Design review of the part built by this model. Coordinates are the model's own, in mm. A direction names the side the tool comes from. Round coordinates to 2 decimals unless told otherwise and drop trailing zeros. Loops run counter-clockwise (first coordinate to the right, second up) from the corner with the lowest first, then second, coordinate; pieces in that order, holes last. Notation, with made-up numbers: (23.25, 48) -> (78.25, 48) arc R28 ccw to (78.25, 72) -> close; hole circle Ø5 at (37.5, 75). An arc over 180 degrees is marked (long way). Use a Markdown table: item, result. Add a question column.
from build123d import *

# Parameters (mm, degrees)
SKETCH_1_W                   = 25
SKETCH_1_H                   = 12
SKETCH_1_W_2                 = 21
SKETCH_1_H_2                 = 8
EXTRUDE_1_DEPTH              = 9
CUT_EXTRUDE_1_DEPTH          = 10
CHAMFER_1_SIZE               = 7
CHAMFER_1_SIZE2              = 1.875644347
HOLE_WIZARD_2_561_AT_2_COUNT = 2
HOLE_WIZARD_2_561_AT_2_PITCH = 5


with BuildPart() as part:
    # Эскиз1 → Бобышка-Вытянуть1 (new body)
    with BuildSketch(Plane.XY):
        with Locations((12.5, 6)):
            Rectangle(SKETCH_1_W, SKETCH_1_H)
        with Locations((12.5, 6)):
            Rectangle(SKETCH_1_W_2, SKETCH_1_H_2, mode=Mode.SUBTRACT)
    extrude(amount=EXTRUDE_1_DEPTH)

    # Эскиз2 → Вырез-Вытянуть1 (cut, through all)
    with BuildSketch(Plane.XY.offset(9)):
        Polygon((18, 10), (18, 12), (0, 12), (0, 0), (19, 0), (19, 2), (2, 2), (2, 10), align=None)
    extrude(amount=-CUT_EXTRUDE_1_DEPTH, mode=Mode.SUBTRACT)

    # Фаска1
    chamfer_1_edges = [part.edges().sort_by_distance(p)[0] for p in [
        (18, 11, 9),
    ]]
    chamfer_1_side = [part.faces().sort_by_distance(p)[0] for p in [
        (18, 11, 4.5),
    ]]
    chamfer(chamfer_1_edges, length=CHAMFER_1_SIZE, length2=CHAMFER_1_SIZE2, reference=chamfer_1_side[0])

    # Эскиз5 → Отверстие обработанное метчиком #2-561 (revolve, cut)
    with BuildSketch(Plane(origin=(21, 0, 2), x_dir=(0, 0, -1), z_dir=(1, 0, 0))):
        Polygon((0, 0), (0, 2), (1.27, 2), (1.0922, 1.8755031), (1.0922, 0.1244969), (1.27, 0), align=None)
    hole_wizard_2_561 = revolve(axis=Axis((21, -6.35, 2), (0, 1, 0)), mode=Mode.SUBTRACT)

    # Отверстие обработанное метчиком #2-561 at 2: Отверстие обработанное метчиком #2-561 ×2
    with Locations(*[(0, 0, i * HOLE_WIZARD_2_561_AT_2_PITCH) for i in range(1, HOLE_WIZARD_2_561_AT_2_COUNT)]):
        add(hole_wizard_2_561, mode=Mode.SUBTRACT)

    # Эскиз6 → Отверстие обработанное метчиком #2-562 (revolve, cut)
    with BuildSketch(Plane(origin=(20.222787252, 12, 4.5), x_dir=(0, 0, 1), z_dir=(1, 0, 0))):
        Polygon((0, 0), (0, 2), (1.27, 2), (1.0922, 1.8755031), (1.0922, 0.1244969), (1.27, 0), align=None)
    revolve(axis=Axis((20.222787252, 18.35, 4.5), (0, -1, 0)), mode=Mode.SUBTRACT)


solid = part.part
1. To check wall thickness, follow probe 1 along Z at (x, y) = (21, 0.85); probe 2 along Y at (x, z) = (19.75, 7.25); probe 3 along X at (y, z) = (1.2, 2). State the ranges of each line that lie inside material, in increasing order. Write a range as from..to.
2. Insertion check: P1, Ø1.5, axis at y = 7.5, z = 3, coming from the -X side; P2, Ø2, axis at y = 1.5, z = 3, coming from the -X side. Each pin has a flat end and moves straight along its axis. Give the tip position at first contact, or say it passes through.
3. Consider section C-C on x = 20.5. Give the number of separate pieces and of enclosed holes in the cut face, plus the area to 3 significant figures.
4. For faces 1 (the face through (21, 10, 3)), 2 (the face through (19, 1, 5)), 3 (the face through (22.066, 0.988, 2.237)), 4 (the face through (22, 12, 4)), 5 (the face through (18.95, 10.99, 5.55)), list the 3-axis set-ups (+Z, -Z, +X, -X, +Y, -Y) from which the entire face can be reached by the end or side of a thin tool; tool diameter is ignored.
5. Consider section D-D on z = 7. State the section outline as (x, y) points.
6. Consider section B-B on y = 9.25. State the section outline as (x, z) points, plus the area to 3 significant figures.
7. Mouldability with a two-part tool opening along X and no side actions: class faces 6 (the face through (23, 6, 4)), 7 (the face through (22.066, 0.988, 7.237)), 8 (the face through (21.29, 11.01, 4.26)), 9 (the face through (21, 2, 4)) as +X half, -X half, draft (parallel to the pull), parting line (faces both ways), or undercut.
8. Consider section A-A on z = 4.5. State the section outline as (x, y) points.
Verdict:
| question | item | result |
|---|---|---|
| 1 | probe 1 | z = 0..0.91, 3.09..5.91, 8.09..9 |
| 1 | probe 2 | y = 0..2, 10..12 |
| 1 | probe 3 | x = 19..19.91, 22.09..25 |
| 2 | P1 | stops at x = 23 |
| 2 | P2 | stops at x = 19 |
| 3 | separate pieces | 5 |
| 3 | enclosed holes | 0 |
| 3 | area | 23.9 mm² |
| 4 | face 1 | +Z, -Z, -X |
| 4 | face 2 | +Z, -Z, -X, -Y |
| 4 | face 3 | -Y |
| 4 | face 4 | +Z, -Z, +X, -X, +Y |
| 4 | face 5 | +Z, -X, +Y |
| 5 | outline | (19, 0) -> (19.73, 0) -> (19.91, 0.12) -> (19.91, 1.88) -> (19.73, 2) -> (19, 2) -> close; (19.34, 10) -> (23, 10) -> (23, 2) -> (22.27, 2) -> (22.09, 1.88) -> (22.09, 0.12) -> (22.27, 0) -> (25, 0) -> (25, 12) -> (19.34, 12) -> close |
| 6 | outline | (23, 0) -> (25, 0) -> (25, 9) -> (23, 9) -> close |
| 6 | area | 18.0 mm² |
| 7 | face 6 | -X half |
| 7 | face 7 | undercut |
| 7 | face 8 | undercut |
| 7 | face 9 | draft |
| 8 | outline | (18.67, 10) -> (18.95, 10) -> (19.13, 10.12) -> (19.13, 11.88) -> (18.95, 12) -> (18.67, 12) -> close; (19, 0) -> (25, 0) -> (25, 12) -> (21.49, 12) -> (21.31, 11.88) -> (21.31, 10.12) -> (21.49, 10) -> (23, 10) -> (23, 2) -> (19, 2) -> close |
